Here's how the part is built. I have some questions about the finished solid (model axes, mm). A direction names the side the tool comes from. Give positions to 0.01 mm unless a question says otherwise; leave off trailing zeros. Loops run counter-clockwise (first coordinate to the right, second up) from the corner with the lowest first, then second, coordinate; pieces in that order, holes last. Notation, with made-up numbers: (-24, -8) - (-9, -8) arc R20 ccw to (-9, -3) - close; hole circle Ø7 at (9, 33). An arc over 180 degrees is marked (long way). Use a Markdown table: item, result.
Autodesk Inventor part; units mm, degrees
ref_plane "Work Plane1" through (-52.6055, -32.2497, -2) normal (0, 0, 1) x (1, 0, 0)
ref_plane "YZ Plane" through (0, 0, 0) normal (1, 0, 0) x (0, 1, 0)
ref_plane "XZ Plane" through (0, 0, 0) normal (0, 1, 0) x (-1, 0, 0)
sketch "Sketch1" plane through (0, 0, 0) normal (0, 0, 1) x (1, 0, 0)
  line L0 (-12.037, -14.2497) -> (-13.9713, -17.6) construction
  line L1 (-13.9713, -17.6) -> (-17.8398, -17.6) construction
  line L2 (-17.8398, -17.6) -> (-19.774, -14.2497) construction
  line L3 (-19.774, -14.2497) -> (-17.8398, -10.8995) construction
  line L4 (-17.8398, -10.8995) -> (-13.9713, -10.8995) construction
  line L5 (-13.9713, -10.8995) -> (-12.037, -14.2497) construction
  circle A0 centre (-15.9055, -14.2497) radius 28.486 construction
  line L6 (-12.1525, -14.2497) -> (-14.029, -17.5)
  line L7 (-14.029, -17.5) -> (-17.782, -17.5)
  line L8 (-17.782, -17.5) -> (-19.6585, -14.2497)
  line L9 (-19.6585, -14.2497) -> (-17.782, -10.9995)
  line L10 (-17.782, -10.9995) -> (-14.029, -10.9995) construction
  line L11 (-14.029, -10.9995) -> (-12.1525, -14.2497)
  line L12 (-15.9055, -10.7856) -> (-18.9055, -15.9818) construction
  line L13 (-18.9055, -15.9818) -> (-12.9055, -15.9818) construction
  line L14 (-12.9055, -15.9818) -> (-15.9055, -10.7856) construction
  line L15 (-15.9055, -11.0856) -> (-18.6457, -15.8318)
  line L16 (-18.6457, -15.8318) -> (-13.1653, -15.8318)
  line L17 (-13.1653, -15.8318) -> (-15.9055, -11.0856)
  point P0 (0, 0)
  dimension "d0" = 0.1
  dimension "d14" = 0.15
extrude "Extrusion1" add sketch "Sketch1" along normal blind 25
sketch "Sketch2" plane through (0, 0, 0) normal (0, 0, 1) x (1, 0, 0)
  circle A0 centre (-15.9055, -14.2497) radius 6 construction
  circle A1 centre (-15.9055, -14.2497) radius 5.5
  point P0 (0, 0)
  dimension "d3" = 0.5
extrude "Extrusion2" add sketch "Sketch2" along normal blind 6
sketch "Sketch3" plane through (-15.9055, -14.2497, 0) normal (0, 0, -1) x (-1, 0, 0)
  circle A0 centre (0, 0) radius 5.5
  point P0 (-15.9055, 14.2497)
ref_plane "Work Plane1" through (-52.6055, -32.2497, -2) normal (0, 0, 1) x (1, 0, 0)
extrude "Extrusion3" add sketch "Sketch3" along normal up to surface (2 mm away)
sketch "Sketch4" plane through (-15.9055, -14.2497, -2) normal (0, 0, -1) x (-1, 0, 0)
  circle A0 centre (0, 0) radius 5.5
  circle A1 centre (0, 0) radius 5.5
  line L0 (-5.2467, -1.65) -> (5.2467, -1.65)
  line L1 (5.2467, -1.65) -> (5.2467, 1.65)
  line L2 (5.2467, 1.65) -> (-5.2467, 1.65)
  line L3 (-5.2467, 1.65) -> (-5.2467, -1.65)
  line L4 (-5.2467, -1.65) -> (5.2467, 1.65) construction
  line L5 (5.2467, -1.65) -> (-5.2467, 1.65) construction
  point P0 (-15.9055, 14.2497)
  dimension "d8" = 3.3
extrude "Extrusion4" add sketch "Sketch4" along normal blind 6.4 contours L1 L0 L3 L2
properties part number "rotor"
(1) Suppose I cut it at C-C on z = -6. Write out the boundary of the cut face in (x, y).
A:
| item | result |
|---|---|
| outline | (-21.15, -15.9) - (-10.66, -15.9) - (-10.66, -12.6) - (-21.15, -12.6) - close |
(2) On a 3-axis mill with a long thin cutter (end or side, diameter ignored), from which of +Z, -Z, +X, -X, +Y, -Y can I reach the whole of each face in a straight line? I mean faces 1 (the face through (-16, -15.832, 15)), 2 (the face through (-10.659, -14, -5)), 3 (the face through (-16, -17, -2)), 4 (the face through (-16, -12.6, -5)). Say none if no direction works.
A:
| item | result |
|---|---|
| face 1 | +Z, +X, -X, -Y |
| face 2 | -Z, +X, +Y, -Y |
| face 3 | -Z, +X, -X, -Y |
| face 4 | -Z, +X, -X, +Y |
(3) If I drill on line 1 (Z direction, x = -15, y = -18.75); line 2 (Z direction, x = -11.25, y = -14); line 3 (X direction, y = -11.25, z = 20), over which ranges is the centre line in solid material (lowest first)?
A:
| item | result |
|---|---|
| line 1 | -2 to 6 |
| line 2 | -8.4 to 6 |
| line 3 | -16 to -15.81 |
(4) Suppose I cut it at B-B on y = -11.5. Write out the boundary of the cut face in (x, z), plus the area to 3 significant figures.
A:
| item | result |
|---|---|
| outline | (-20.67, -2) - (-11.14, -2) - (-11.14, 6) - (-15.67, 6) - (-15.67, 25) - (-16.14, 25) - (-16.14, 6) - (-20.67, 6) - close |
| area | 85.3 mm2 |
(5) Suppose I cut it at D-D on x = -20.25. Write out the boundary of the cut face in (y, z).
A:
| item | result |
|---|---|
| outline | (-17.62, -2) - (-15.9, -2) - (-15.9, -8.4) - (-12.6, -8.4) - (-12.6, -2) - (-10.88, -2) - (-10.88, 6) - (-17.62, 6) - close |
(6) Will these pins go through, and if not, where does the flat tip stop? pin 1 (1.9 mm diameter, centred on x = -16, y = -11, fed in from -Z); pin 2 (1.6 mm diameter, centred on y = -15, z = -4.5, fed in from -X); pin 3 (2.5 mm diameter, centred on y = -15, z = -6.5, fed in from +X).
A:
| item | result |
|---|---|
| pin 1 | z = -2 |
| pin 2 | x = -21.15 |
| pin 3 | x = -10.66 |
(7) Suppose I cut it at A-A on x = -16.25. Write out the boundary of the cut face in (y, z), plus the area to 3 significant figures.
A:
| item | result |
|---|---|
| outline | (-19.74, -2) - (-15.9, -2) - (-15.9, -8.4) - (-12.6, -8.4) - (-12.6, -2) - (-8.76, -2) - (-8.76, 6) - (-11.68, 6) - (-11.68, 25) - (-15.83, 25) - (-15.83, 6) - (-19.74, 6) - close |
| area | 188 mm2 |
